Design review of the part built by this model. Coordinates are the model's own, in mm. Face numbers are marked on the shaded views. A direction names the side the tool comes from. Give positions to 0.01 mm unless a question says otherwise; leave off trailing zeros. Write each loop counter-clockwise with the first axis right and the second up, starting at its lowest first coordinate (ties: lowest second). Pieces come first, ordered by that corner, then holes. Notation, with made-up numbers: M -38.5,89.25 L -21.5,89.25 A34 cw -21.5,119.25 Z; hole C 48.25,18 d7. An arc over 180 degrees is marked long. One line per item, written item: value. Start each with the question number.
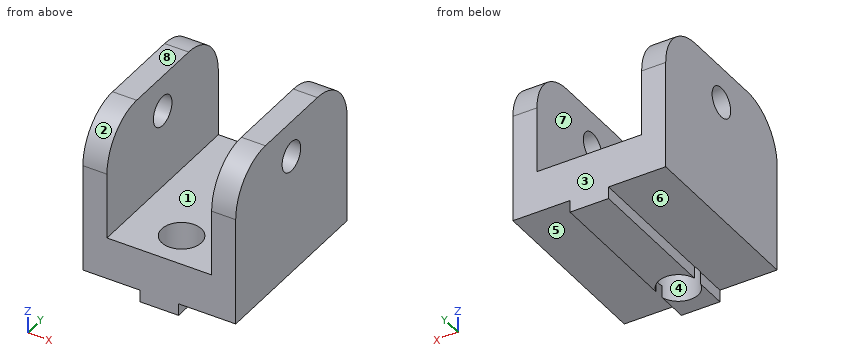
```python
from build123d import *

# Parameters (mm, degrees)
F0_R     = 2.5
F1_DEPTH = 25.4
F2_W     = 17.4
F2_H     = 38.590171
F3_DEPTH = 19
F4_W     = 6.4
F4_H     = 30
F5_DEPTH = 2
F6_R     = 3.3
F7_DEPTH = 10


with BuildPart() as f1:
    # F0 (on Right) → F1 (new body)
    with BuildSketch(Plane.YZ):
        with BuildLine():
            Line((7, 26), (-7, 26))
            ThreePointArc((-7, 26), (-12.656854, 23.656854), (-15, 18))
            Line((-15, 18), (-15, 0))
            Line((-15, 0), (15, 0))
            Line((15, 0), (15, 18))
            ThreePointArc((15, 18), (12.656854, 23.656854), (7, 26))
        make_face()
        with Locations((0, 20)):
            Circle(F0_R, mode=Mode.SUBTRACT)
    extrude(amount=F1_DEPTH)

    # F2 (on face) → F3 (cut)
    with BuildSketch(Plane.XY.offset(26)):
        with Locations((12.7, -0.404529)):
            Rectangle(F2_W, F2_H)
    extrude(amount=-F3_DEPTH, mode=Mode.SUBTRACT)

    # F4 (on face) → F5 (join)
    with BuildSketch(Plane(origin=(0, 0, 0), x_dir=(1, 0, 0), z_dir=(0, 0, -1))):
        with Locations((12.7, 0)):
            Rectangle(F4_W, F4_H)
    extrude(amount=F5_DEPTH)

    # F6 (on face) → F7 (cut)
    with BuildSketch(Plane.XY.offset(7)):
        with Locations((12.7, -9)):
            Circle(F6_R)
    extrude(amount=-F7_DEPTH, mode=Mode.SUBTRACT)


solid = f1.part
```
Q1. Take a section at D-D, the plane z = 21.25. Give the boundary of the cut face in (x, y), then the cut area to 3 significant figures.
Q2. Take a section at C-C, the plane x = 12.7. Give the boundary of the cut face in (y, z).
Q3. For P1, Ø3, axis at x = 21, y = -0.5, coming from the -Z side; P2, Ø4, axis at x = 16, y = 9.5, coming from the +Z side; P3, Ø4, axis at x = 22.5, z = 22, coming from the +Y side; P4, Ø4.5, axis at y = 0, z = 20, coming from the +X side, all flat-tipped, find the tip position at first contact; note any pin that passes through.
Q4. Take a section at A-A, the plane y = 2. Give the boundary of the cut face in (x, z).
Q5. The part is to be moulded in two halves that separate along Y. For the marked faces 1, 2, 3 and 4, say which applies: pulls with the +Y half, pulls with the -Y half, needs draft (parallel to the pull), parting line crosses it, or undercut.
Q6. Take a section at B-B, the plane z = 11.75. Give the boundary of the cut face in (x, y).
Q7. Machinability: for the marked faces 5, 6, 7 and 8, which of the approach directions +Z, -Z, +X, -X, +Y, -Y give a long, thin tool a straight path to every point of the face, cutting with its end or side? Answer none if there is none.
Q8. Wall thickness on line 1 (X direction, y = 7.75, z = 20.75); line 2 (Z direction, x = 1.85, y = 0); line 3 (X direction, y = -9, z = 5.25): over which ranges is each line inside the solid? List them lowest first. Write a range as from..to.
Results list:
1. outline: M 0,-14.31 L 4,-14.31 L 4,-2.17 L 0,-2.17 Z; M 0,2.17 L 4,2.17 L 4,14.31 L 0,14.31 Z; M 21.4,-14.31 L 25.4,-14.31 L 25.4,-2.17 L 21.4,-2.17 Z; M 21.4,2.17 L 25.4,2.17 L 25.4,14.31 L 21.4,14.31 Z
1. area: 194 mm^2
2. outline: M -15,-2 L -12.3,-2 L -12.3,7 L -15,7 Z; M -5.7,-2 L 15,-2 L 15,7 L -5.7,7 Z
3. P1: stops at z = 0
3. P2: stops at z = 7
3. P3: stops at y = 14.75
3. P4: passes through
4. outline: M 0,0 L 9.5,0 L 9.5,-2 L 15.9,-2 L 15.9,0 L 25.4,0 L 25.4,18.5 L 21.4,18.5 L 21.4,7 L 4,7 L 4,18.5 L 0,18.5 Z; M 0,21.5 L 4,21.5 L 4,26 L 0,26 Z; M 21.4,21.5 L 25.4,21.5 L 25.4,26 L 21.4,26 Z
5. face 1: needs draft
5. face 2: pulls with the -Y half
5. face 3: pulls with the +Y half
5. face 4: undercut
6. outline: M 0,-15 L 4,-15 L 4,15 L 0,15 Z; M 21.4,-15 L 25.4,-15 L 25.4,15 L 21.4,15 Z
7. face 5: -Z, +X, +Y, -Y
7. face 6: -Z, -X, +Y, -Y
7. face 7: +Z, +Y, -Y
7. face 8: +Z, +X, -X, +Y, -Y
8. line 1: x = 0..4, 21.4..25.4
8. line 2: z = 0..17.5, 22.5..26
8. line 3: x = 0..9.4, 16..25.4
